Could you check a few things on this model? Use its own coordinates, in mm. Round coordinates to 2 decimals unless told otherwise and drop trailing zeros. Loops run counter-clockwise (first coordinate to the right, second up) from the corner with the lowest first, then second, coordinate; pieces in that order, holes last. Notation, with made-up numbers: (73, 33.5) -> (103, 33.5) arc R18 ccw to (103, 65.5) -> close; hole circle Ø2 at (56, -33.75). An arc over 180 degrees is marked (long way). One line per item, written item: value.
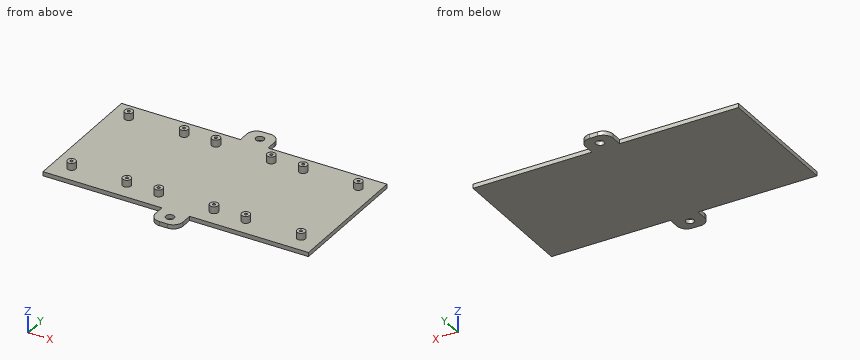
Autodesk Fusion 360 part; units mm, degrees
sketch "Sketch1" plane through (0, 0, 0) normal (0, 0, 1) x (1, 0, 0)
  line L0 (0, 0) -> (192, 0)
  line L1 (192, 0) -> (192, 96)
  line L2 (192, 96) -> (0, 96)
  line L3 (0, 96) -> (0, 0)
  dimension "d1" = 192
  dimension "d2" = 96
extrude "Extrude1" add sketch "Sketch1" along normal blind 3
sketch "Sketch3" plane through (0, 0, 3) normal (0, 0, 1) x (-1, 0, 0)
  line L0 (0, -96) -> (0, 0)
  line L1 (0, 0) -> (-192, 0)
  line L2 (-192, 0) -> (-192, -96)
  line L3 (-192, -96) -> (0, -96)
  line L4 (-3, -93) -> (-63, -93)
  line L5 (-63, -93) -> (-63, -3)
  line L6 (-63, -3) -> (-3, -3)
  line L7 (-3, -3) -> (-3, -93)
  circle A0 centre (-13, -83) radius 1
  circle A1 centre (-53, -83) radius 1
  circle A2 centre (-13, -13) radius 1
  circle A3 centre (-53, -13) radius 1
  circle A4 centre (-13, -83) radius 3
  circle A5 centre (-53, -83) radius 3
  circle A6 centre (-13, -13) radius 3
  circle A7 centre (-53, -13) radius 3
  dimension "d7" = 60
  dimension "d8" = 90
  dimension "d9" = 3
  dimension "d10" = 3
  dimension "d11" = 2
  dimension "d12" = 10
  dimension "d13" = 10
  dimension "d14" = 2
  dimension "d15" = 10
  dimension "d16" = 10
  dimension "d17" = 2
  dimension "d18" = 10
  dimension "d19" = 10
  dimension "d20" = 2
  dimension "d21" = 10
  dimension "d22" = 10
  dimension "d23" = 6
  dimension "d24" = 6
  dimension "d25" = 6
  dimension "d26" = 6
extrude "Extrude2" add sketch "Sketch3" along normal blind 5 contours A4 | A5 | A6 | A7
sketch "Sketch4" plane through (0, 0, 3) normal (0, 0, 1) x (-1, 0, 0)
  circle A0 centre (-13, -83) radius 3
  circle A1 centre (-53, -83) radius 3
  line L0 (0, -96) -> (0, 0)
  line L1 (0, 0) -> (-192, 0)
  line L2 (-192, 0) -> (-192, -96)
  line L3 (-192, -96) -> (0, -96)
  circle A2 centre (-53, -13) radius 3
  circle A3 centre (-13, -13) radius 3
  line L4 (-66, -3) -> (-66, -93)
  circle A4 centre (-116, -13) radius 3
  line L5 (-66, -93) -> (-126, -93)
  line L6 (-126, -3) -> (-66, -3)
  circle A5 centre (-76, -13) radius 3
  circle A6 centre (-76, -83) radius 3
  line L7 (-126, -93) -> (-126, -3)
  circle A7 centre (-76, -13) radius 1
  circle A8 centre (-116, -83) radius 3
  circle A9 centre (-116, -13) radius 1
  line L8 (-63, -96) -> (-63, 0)
  circle A10 centre (-116, -83) radius 1
  circle A11 centre (-76, -83) radius 1
  line L9 (-129, -3) -> (-129, -93)
  circle A12 centre (-179, -13) radius 3
  line L10 (-129, -93) -> (-189, -93)
  line L11 (-189, -3) -> (-129, -3)
  circle A13 centre (-139, -13) radius 3
  circle A14 centre (-139, -83) radius 3
  line L12 (-189, -93) -> (-189, -3)
  circle A15 centre (-139, -13) radius 1
  circle A16 centre (-179, -83) radius 3
  circle A17 centre (-179, -13) radius 1
  line L13 (-126, -96) -> (-126, 0)
  circle A18 centre (-179, -83) radius 1
  circle A19 centre (-139, -83) radius 1
  point P0 (-63, 0)
  point P1 (-126, 0)
  dimension "d29" = 60
  dimension "d30" = 90
  dimension "d31" = 3
  dimension "d32" = 2
  dimension "d33" = 10
  dimension "d34" = 10
  dimension "d35" = 2
  dimension "d36" = 10
  dimension "d37" = 10
  dimension "d38" = 2
  dimension "d39" = 10
  dimension "d40" = 10
  dimension "d41" = 2
  dimension "d42" = 10
  dimension "d43" = 10
  dimension "d44" = 6
  dimension "d45" = 6
  dimension "d46" = 6
  dimension "d47" = 6
  dimension "d48" = 60
  dimension "d49" = 90
  dimension "d50" = 3
  dimension "d51" = 2
  dimension "d52" = 10
  dimension "d53" = 10
  dimension "d54" = 2
  dimension "d55" = 10
  dimension "d56" = 10
  dimension "d57" = 2
  dimension "d58" = 10
  dimension "d59" = 10
  dimension "d60" = 2
  dimension "d61" = 10
  dimension "d62" = 10
  dimension "d63" = 6
  dimension "d64" = 6
  dimension "d65" = 6
  dimension "d66" = 6
extrude "Extrude3" add sketch "Sketch4" along normal blind 5 contours A4 | A5 | A6 | A8 | A12 | A13 | A14 | A16
sketch "Sketch5" plane through (0, 0, 3) normal (0, 0, 1) x (-1, 0, 0)
  circle A0 centre (-179, -83) radius 3
  circle A1 centre (-179, -13) radius 3
  circle A2 centre (-139, -83) radius 3
  circle A3 centre (-139, -13) radius 3
  circle A4 centre (-13, -83) radius 3
  circle A5 centre (-53, -83) radius 3
  line L0 (0, -96) -> (0, 0)
  line L1 (0, 0) -> (-192, 0)
  line L2 (-192, 0) -> (-192, -96)
  line L3 (-192, -96) -> (0, -96)
  circle A6 centre (-53, -13) radius 3
  circle A7 centre (-13, -13) radius 3
  circle A8 centre (-116, -83) radius 3
  circle A9 centre (-116, -13) radius 3
  circle A10 centre (-76, -83) radius 3
  circle A11 centre (-76, -13) radius 3
  line L4 (-86, -96) -> (-106, -96)
  line L5 (-106, -96) -> (-106, -104)
  line L6 (-99, -111) -> (-93, -111)
  line L7 (-86, -104) -> (-86, -96)
  circle A12 centre (-96, -103) radius 3
  arc A13 (-93, -111) -> (-86, -104) centre (-93, -104) ccw
  arc A14 (-106, -104) -> (-99, -111) centre (-99, -104) ccw
  line L8 (0, -48) -> (-192, -48)
  arc A15 (-86, 8) -> (-93, 15) centre (-93, 8) ccw
  arc A16 (-99, 15) -> (-106, 8) centre (-99, 8) ccw
  line L9 (-86, 0) -> (-106, 0)
  line L10 (-86, 8) -> (-86, 0)
  line L11 (-106, 0) -> (-106, 8)
  circle A17 centre (-96, 7) radius 3
  line L12 (-99, 15) -> (-93, 15)
  line L13 (-192, 0) -> (0, 0)
  point P0 (-86, -111)
  point P1 (-86, 15)
  dimension "d69" = 20
  dimension "d70" = 15
  dimension "d71" = 6
  dimension "d72" = 7
  dimension "d73" = 7
extrude "Extrude4" add sketch "Sketch5" against normal blind 3 contours L3 L4 L5 L6 L7 A13 A14 | L1 A15 A16 L9 L10 L11 L12 L13
(1) If we section it at A-A, the plane x = 96: Please give me the cut outline in (y, z).
Recorded:
outline: (-15, 0) -> (-10, 0) -> (-10, 3) -> (-15, 3) -> close; (-4, 0) -> (100, 0) -> (100, 3) -> (-4, 3) -> close; (106, 0) -> (111, 0) -> (111, 3) -> (106, 3) -> close
(2) If we section it at B-B, the plane z = 1.75: Please give me the cut outline in (x, y).
Recorded:
outline: (0, 0) -> (86, 0) -> (86, -8) arc R7 ccw to (93, -15) -> (99, -15) arc R7 ccw to (106, -8) -> (106, 0) -> (192, 0) -> (192, 96) -> (106, 96) -> (106, 104) arc R7 ccw to (99, 111) -> (93, 111) arc R7 ccw to (86, 104) -> (86, 96) -> (0, 96) -> close; hole circle Ø6 at (96, -7); hole circle Ø6 at (96, 103)
(3) I'm going to push flat-ended pins straight in: pin 1 Ø5 at (x, y) = (135.5, -0.5) entering from -Z; pin 2 Ø0.9 at (y, z) = (101.5, 1.5) entering from +X; pin 3 Ø1.5 at (x, z) = (171.5, 1.5) entering from +Y; pin 4 Ø3.5 at (y, z) = (101, 2) entering from -X. Where does each tip first touch, or does it pass through?
Recorded:
pin 1: z = 0
pin 2: x = 106
pin 3: y = 96
pin 4: x = 86
(4) If we section it at C-C, the plane y = 72: Please give me the cut outline in (x, z).
Recorded:
outline: (0, 0) -> (192, 0) -> (192, 3) -> (0, 3) -> close
(5) If I drill on L1, parallel to Y at x = 76, z = 6.75; L2, parallel to Z at x = 172.5, y = 66.5; L3, parallel to Y at x = 16.5, z = 2.5, over which ranges is the centre line in solid material (lowest first)?
Recorded:
L1: 10 to 12, 14 to 16, 80 to 82, 84 to 86
L2: 0 to 3
L3: 0 to 96
(6) If we section it at D-D, the plane x = 147: Please give me the cut outline in (y, z), then the cut area to 3 significant figures.
Recorded:
outline: (0, 0) -> (96, 0) -> (96, 3) -> (0, 3) -> close
area: 288 mm²
